Verification items for the finished model (mm, model axes). Face numbers are marked on the shaded views. Give positions to 0.01 mm unless a question says otherwise; leave off trailing zeros. Write each loop counter-clockwise with the first axis right and the second up, starting at its lowest first coordinate (ties: lowest second). Pieces come first, ordered by that corner, then holes. Notation, with made-up numbers: M 29.25,47.5 L 43.25,47.5 A17 cw 43.25,68.5 Z; hole C 51,9 d8. An arc over 180 degrees is marked long. Write item = value, one per line.
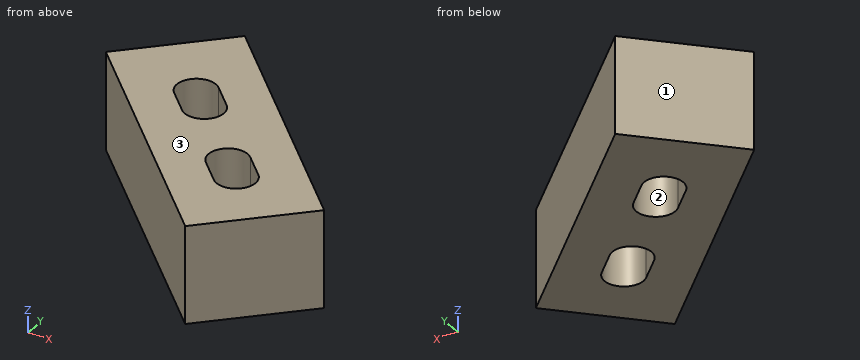
Autodesk Inventor part; units mm, degrees
ref_plane "YZ Plane" through (0, 0, 0) normal (1, 0, 0) x (0, 1, 0)
ref_plane "XZ Plane" through (0, 0, 0) normal (0, 1, 0) x (-1, 0, 0)
ref_plane "XY Plane" through (0, 0, 0) normal (0, 0, 1) x (1, 0, 0)
sketch "Sketch1" plane through (0, 0, 0) normal (0, 0, 1) x (1, 0, 0)
  line L0 (7.0711, 21.2132) -> (20.3934, 34.5355)
  line L1 (61, 1) -> (41.6066, 20.3934)
  line L2 (61, 1) -> (725, 1)
  line L3 (725, 1) -> (725, 26)
  line L4 (725, 26) -> (720, 31)
  line L5 (720, 31) -> (437.7615, 31)
  arc A0 (434.226, 32.4645) -> (437.7615, 31) centre (437.7615, 36) ccw
  line L6 (434.226, 32.4645) -> (32.4645, 434.226)
  arc A1 (31, 437.7615) -> (32.4645, 434.226) centre (36, 437.7615) ccw
  line L7 (31, 437.7615) -> (31, 720)
  line L8 (31, 720) -> (26, 725)
  line L9 (26, 725) -> (1, 725)
  line L10 (1, 725) -> (1, 61)
  line L11 (20.3934, 41.6066) -> (1, 61)
  arc A2 (20.3934, 34.5355) -> (20.3934, 41.6066) centre (16.8579, 38.0711) ccw
  line L12 (7.0711, 21.2132) -> (20.3934, 34.5355)
  line L13 (21.2132, 7.0711) -> (7.0711, 21.2132)
  line L14 (34.5355, 20.3934) -> (21.2132, 7.0711)
  arc A3 (41.6066, 20.3934) -> (34.5355, 20.3934) centre (38.0711, 16.8579) ccw
  circle A4 centre (15, 600) radius 3.2
  circle A5 centre (200, 15) radius 3.2
  circle A6 centre (600, 15) radius 3.2
  line L15 (252.9319, 164.2611) -> (377.6575, 39.5355)
  arc A7 (374.1219, 31) -> (377.6575, 39.5355) centre (374.1219, 36) ccw
  line L16 (374.1219, 31) -> (82.5685, 31)
  arc A8 (79.033, 32.4645) -> (82.5685, 31) centre (82.5685, 36) ccw
  line L17 (79.033, 32.4645) -> (32.4645, 79.033)
  arc A9 (31, 82.5685) -> (32.4645, 79.033) centre (36, 82.5685) ccw
  line L18 (31, 82.5685) -> (31, 374.1219)
  arc A10 (39.5355, 377.6575) -> (31, 374.1219) centre (36, 374.1219) ccw
  line L19 (39.5355, 377.6575) -> (164.2611, 252.9319)
  arc A11 (162.7002, 244.8028) -> (164.2611, 252.9319) centre (160.7256, 249.3963) ccw
  arc A12 (162.7002, 244.8028) -> (244.8028, 162.7002) centre (187.3833, 187.3833) ccw
  arc A13 (252.9319, 164.2611) -> (244.8028, 162.7002) centre (249.3963, 160.7256) ccw
  circle A14 centre (15, 200) radius 3.2
  line L20 (-61, -1) -> (-41.6066, -20.3934)
  line L21 (-61, -1) -> (-725, -1)
  line L22 (-725, -1) -> (-725, -26)
  line L23 (-725, -26) -> (-720, -31)
  line L24 (-720, -31) -> (-437.7615, -31)
  arc A15 (-434.226, -32.4645) -> (-437.7615, -31) centre (-437.7615, -36) ccw
  line L25 (-434.226, -32.4645) -> (-32.4645, -434.226)
  arc A16 (-31, -437.7615) -> (-32.4645, -434.226) centre (-36, -437.7615) ccw
  line L26 (-31, -437.7615) -> (-31, -720)
  line L27 (-31, -720) -> (-26, -725)
  line L28 (-26, -725) -> (-1, -725)
  line L29 (-1, -725) -> (-1, -61)
  line L30 (-20.3934, -41.6066) -> (-1, -61)
  arc A17 (-20.3934, -34.5355) -> (-20.3934, -41.6066) centre (-16.8579, -38.0711) ccw
  line L31 (-7.0711, -21.2132) -> (-20.3934, -34.5355)
  line L32 (-21.2132, -7.0711) -> (-7.0711, -21.2132)
  line L33 (-34.5355, -20.3934) -> (-21.2132, -7.0711)
  arc A18 (-41.6066, -20.3934) -> (-34.5355, -20.3934) centre (-38.0711, -16.8579) ccw
  circle A19 centre (-15, -600) radius 3.2
  circle A20 centre (-200, -15) radius 3.2
  circle A21 centre (-600, -15) radius 3.2
  line L34 (-252.9319, -164.2611) -> (-377.6575, -39.5355)
  arc A22 (-374.1219, -31) -> (-377.6575, -39.5355) centre (-374.1219, -36) ccw
  line L35 (-374.1219, -31) -> (-82.5685, -31)
  arc A23 (-79.033, -32.4645) -> (-82.5685, -31) centre (-82.5685, -36) ccw
  line L36 (-79.033, -32.4645) -> (-32.4645, -79.033)
  arc A24 (-31, -82.5685) -> (-32.4645, -79.033) centre (-36, -82.5685) ccw
  line L37 (-31, -82.5685) -> (-31, -374.1219)
  arc A25 (-39.5355, -377.6575) -> (-31, -374.1219) centre (-36, -374.1219) ccw
  line L38 (-39.5355, -377.6575) -> (-164.2611, -252.9319)
  arc A26 (-162.7002, -244.8028) -> (-164.2611, -252.9319) centre (-160.7256, -249.3963) ccw
  arc A27 (-162.7002, -244.8028) -> (-244.8028, -162.7002) centre (-187.3833, -187.3833) ccw
  arc A28 (-252.9319, -164.2611) -> (-244.8028, -162.7002) centre (-249.3963, -160.7256) ccw
  circle A29 centre (-15, -200) radius 3.2
  line L39 (-1, 61) -> (-20.3934, 41.6066)
  line L40 (-1, 61) -> (-1, 725)
  line L41 (-1, 725) -> (-26, 725)
  line L42 (-26, 725) -> (-31, 720)
  line L43 (-31, 720) -> (-31, 437.7615)
  arc A30 (-32.4645, 434.226) -> (-31, 437.7615) centre (-36, 437.7615) ccw
  line L44 (-32.4645, 434.226) -> (-434.226, 32.4645)
  arc A31 (-437.7615, 31) -> (-434.226, 32.4645) centre (-437.7615, 36) ccw
  line L45 (-437.7615, 31) -> (-720, 31)
  line L46 (-720, 31) -> (-725, 26)
  line L47 (-725, 26) -> (-725, 1)
  line L48 (-725, 1) -> (-61, 1)
  line L49 (-41.6066, 20.3934) -> (-61, 1)
  arc A32 (-34.5355, 20.3934) -> (-41.6066, 20.3934) centre (-38.0711, 16.8579) ccw
  line L50 (-21.2132, 7.0711) -> (-34.5355, 20.3934)
  line L51 (-7.0711, 21.2132) -> (-21.2132, 7.0711)
  line L52 (-20.3934, 34.5355) -> (-7.0711, 21.2132)
  arc A33 (-20.3934, 41.6066) -> (-20.3934, 34.5355) centre (-16.8579, 38.0711) ccw
  circle A34 centre (-600, 15) radius 3.2
  circle A35 centre (-15, 200) radius 3.2
  circle A36 centre (-15, 600) radius 3.2
  line L53 (-164.2611, 252.9319) -> (-39.5355, 377.6575)
  arc A37 (-31, 374.1219) -> (-39.5355, 377.6575) centre (-36, 374.1219) ccw
  line L54 (-31, 374.1219) -> (-31, 82.5685)
  arc A38 (-32.4645, 79.033) -> (-31, 82.5685) centre (-36, 82.5685) ccw
  line L55 (-32.4645, 79.033) -> (-79.033, 32.4645)
  arc A39 (-82.5685, 31) -> (-79.033, 32.4645) centre (-82.5685, 36) ccw
  line L56 (-82.5685, 31) -> (-374.1219, 31)
  arc A40 (-377.6575, 39.5355) -> (-374.1219, 31) centre (-374.1219, 36) ccw
  line L57 (-377.6575, 39.5355) -> (-252.9319, 164.2611)
  arc A41 (-244.8028, 162.7002) -> (-252.9319, 164.2611) centre (-249.3963, 160.7256) ccw
  arc A42 (-244.8028, 162.7002) -> (-162.7002, 244.8028) centre (-187.3833, 187.3833) ccw
  arc A43 (-164.2611, 252.9319) -> (-162.7002, 244.8028) centre (-160.7256, 249.3963) ccw
  circle A44 centre (-200, 15) radius 3.2
  line L58 (1, -61) -> (20.3934, -41.6066)
  line L59 (1, -61) -> (1, -725)
  line L60 (1, -725) -> (26, -725)
  line L61 (26, -725) -> (31, -720)
  line L62 (31, -720) -> (31, -437.7615)
  arc A45 (32.4645, -434.226) -> (31, -437.7615) centre (36, -437.7615) ccw
  line L63 (32.4645, -434.226) -> (434.226, -32.4645)
  arc A46 (437.7615, -31) -> (434.226, -32.4645) centre (437.7615, -36) ccw
  line L64 (437.7615, -31) -> (720, -31)
  line L65 (720, -31) -> (725, -26)
  line L66 (725, -26) -> (725, -1)
  line L67 (725, -1) -> (61, -1)
  line L68 (41.6066, -20.3934) -> (61, -1)
  arc A47 (34.5355, -20.3934) -> (41.6066, -20.3934) centre (38.0711, -16.8579) ccw
  line L69 (21.2132, -7.0711) -> (34.5355, -20.3934)
  line L70 (7.0711, -21.2132) -> (21.2132, -7.0711)
  line L71 (20.3934, -34.5355) -> (7.0711, -21.2132)
  arc A48 (20.3934, -41.6066) -> (20.3934, -34.5355) centre (16.8579, -38.0711) ccw
  circle A49 centre (600, -15) radius 3.2
  circle A50 centre (15, -200) radius 3.2
  circle A51 centre (15, -600) radius 3.2
  line L72 (164.2611, -252.9319) -> (39.5355, -377.6575)
  arc A52 (31, -374.1219) -> (39.5355, -377.6575) centre (36, -374.1219) ccw
  line L73 (31, -374.1219) -> (31, -82.5685)
  arc A53 (32.4645, -79.033) -> (31, -82.5685) centre (36, -82.5685) ccw
  line L74 (32.4645, -79.033) -> (79.033, -32.4645)
  arc A54 (82.5685, -31) -> (79.033, -32.4645) centre (82.5685, -36) ccw
  line L75 (82.5685, -31) -> (374.1219, -31)
  arc A55 (377.6575, -39.5355) -> (374.1219, -31) centre (374.1219, -36) ccw
  line L76 (377.6575, -39.5355) -> (252.9319, -164.2611)
  arc A56 (244.8028, -162.7002) -> (252.9319, -164.2611) centre (249.3963, -160.7256) ccw
  arc A57 (244.8028, -162.7002) -> (162.7002, -244.8028) centre (187.3833, -187.3833) ccw
  arc A58 (164.2611, -252.9319) -> (162.7002, -244.8028) centre (160.7256, -249.3963) ccw
  circle A59 centre (200, -15) radius 3.2
  line L77 (-8.1812, 19.7495) -> (8.1812, 19.7495)
  line L78 (19.7495, 8.1812) -> (8.1812, 19.7495)
  line L79 (19.7495, 8.1812) -> (19.7495, -8.1812)
  line L80 (13.9654, -13.9654) -> (19.7495, -8.1812)
  line L81 (5.6569, -5.6569) -> (13.9654, -13.9654)
  arc A60 (5.6569, -5.6569) -> (-5.6569, 5.6569) centre (0, 0) ccw
  line L82 (-13.9654, 13.9654) -> (-5.6569, 5.6569)
  line L83 (-8.1812, 19.7495) -> (-13.9654, 13.9654)
  line L84 (8.1812, -19.7495) -> (-8.1812, -19.7495)
  line L85 (-19.7495, -8.1812) -> (-8.1812, -19.7495)
  line L86 (-19.7495, -8.1812) -> (-19.7495, 8.1812)
  line L87 (-13.9654, 13.9654) -> (-19.7495, 8.1812)
  line L88 (-5.6569, 5.6569) -> (-13.9654, 13.9654)
  arc A61 (-5.6569, 5.6569) -> (5.6569, -5.6569) centre (0, 0) ccw
  line L89 (13.9654, -13.9654) -> (5.6569, -5.6569)
  line L90 (8.1812, -19.7495) -> (13.9654, -13.9654)
  line L91 (-4.0659, 18.208) -> (-18.208, 4.0659)
  line L92 (-18.208, 4.0659) -> (-53.5633, 39.4212)
  line L93 (-18.208, 4.0659) -> (31.792, 4.0659) construction
  line L94 (-4.0659, 18.208) -> (-39.4212, 53.5633)
  line L95 (-45.1904, 45.1904) -> (-11.1369, 11.1369) construction
  line L96 (-19.4454, 19.4454) -> (-22.981, 22.981) construction
  line L97 (-17.1827, 21.7082) -> (-20.7182, 25.2437)
  line L98 (-25.2437, 20.7182) -> (-21.7082, 17.1827)
  arc A62 (-21.7082, 17.1827) -> (-17.1827, 21.7082) centre (-19.4454, 19.4454) ccw
  arc A63 (-20.7182, 25.2437) -> (-25.2437, 20.7182) centre (-22.981, 22.981) ccw
  line L99 (-33.5876, 33.5876) -> (-37.1231, 37.1231) construction
  line L100 (-31.3248, 35.8503) -> (-34.8604, 39.3858)
  line L101 (-39.3858, 34.8604) -> (-35.8503, 31.3248)
  arc A64 (-35.8503, 31.3248) -> (-31.3248, 35.8503) centre (-33.5876, 33.5876) ccw
  arc A65 (-34.8604, 39.3858) -> (-39.3858, 34.8604) centre (-37.1231, 37.1231) ccw
  line L102 (-53.5633, 39.4212) -> (-39.4212, 53.5633)
  point P0 (0, 0)
  point P1 (-21.2132, 21.2132)
  point P2 (-35.3553, 35.3553)
extrude "Extrusion2" add sketch "Sketch1" along normal blind 15.875 contours L52 L51 L50 L92 L102 L94 | L94 L77 L83 L87 L86 L92 L51 | L94 L91 L82 L83 L77 | L86 L87 L82 L91 L92
properties part number "Conduit-brace"
1) Cross-section at C-C on x = -34. Record the boundary of the cut face in (y, z) (3 decimals).
From the geometry:
outline = M 19.858,0 L 30.414,0 L 30.414,15.875 L 19.858,15.875 Z; M 38.525,0 L 48.142,0 L 48.142,15.875 L 38.525,15.875 Z
2) Draft check along Y on the marked faces 1, 2 and 3. Enter one of: +Y half, -Y half, draft (parallel to the pull), parting line (faces both ways), or undercut.
From the geometry:
face_1 = +Y half
face_2 = undercut
face_3 = draft
3) Cross-section at D-D on y = 27. Record the boundary of the cut face in (x, z) (3 decimals), plus the area to 3 significant figures.
From the geometry:
outline = M -41.142,0 L -12.858,0 L -12.858,15.875 L -41.142,15.875 Z
area = 449 mm^2
4) Cross-section at B-B on y = 32. Record the boundary of the cut face in (x, z) (3 decimals).
From the geometry:
outline = M -46.142,0 L -36.525,0 L -36.525,15.875 L -46.142,15.875 Z; M -30.809,0 L -17.858,0 L -17.858,15.875 L -30.809,15.875 Z
5) Depth check by flat-ended pin: P1, Ø2, axis at x = -25, z = 5.5, coming from the -Y side; P2, Ø4, axis at x = -15, z = 10, coming from the +Y side; P3, Ø4, axis at y = 47, z = 6.5, coming from the +X side. Enter the tip coordinate at first touch or a pass-through.
From the geometry:
P1 = 9.86
P2 = 31.14
P3 = -30.86
6) Cross-section at A-A on z = 14. Record the boundary of the cut face in (x, y).
From the geometry:
outline = M -53.56,39.42 L -18.21,4.07 L -4.07,18.21 L -39.42,53.56 Z; hole M -39.39,34.86 L -35.85,31.32 A3.2 ccw -31.32,35.85 L -34.86,39.39 A3.2 ccw Z; hole M -25.24,20.72 L -21.71,17.18 A3.2 ccw -17.18,21.71 L -20.72,25.24 A3.2 ccw Z
7) Material ranges on probe 1 along X at (y, z) = (16.5, 4); probe 2 along X at (y, z) = (24, 11); probe 3 along Y at (x, z) = (-36.5, 8.5), recorded low to high. Write a range as from..to.
From the geometry:
probe_1 = -30.64..-20.7, -18.19..-5.77
probe_2 = -38.14..-26.01, -19.47..-9.86
probe_3 = 22.36..31.97, 40.26..50.64
